Autodesk Fusion 360 part; units mm, degrees
box "BoxPrimitive1" add length 25 width 40 height 25 placed x (0, 0, -1) y (-1, 0, 0) z (0, 1, 0) at (40, 0, 0)
hole "Hole1" at (20, 25, -12.5) direction (0, -1, 0) diameter 8.8 depth 18 tip angle 180
sketch "Sketch2" plane through (40, 0, 0) normal (1, 0, 0) x (0, 0, -1)
  line L0 (0, 25) -> (0, 0)
  line L1 (0, 0) -> (25, 0)
  line L2 (25, 0) -> (25, 25)
  line L3 (25, 25) -> (0, 25)
  line L4 (12.5, 25) -> (12.5, 7) construction
  point P0 (12.5, 9)
  dimension "d9" = 18
  dimension "d10" = 2
hole "Hole2" at (40, 9, -12.5) direction (-1, 0, 0) diameter 2 end through all
hole "Hole3" at (40, 9, -12.5) direction (-1, 0, 0) diameter 6.8 depth 14 tip angle 180
hole "Hole5" at (40, 9, -12.5) direction (-1, 0, 0) diameter 7.2 depth 7.5 tip angle 180
ref_plane "WorkPlane1" through (20, 12.5, -12.5) normal (-1, 0, 0) x (0, 1, 0)
mirror "Mirror1" about plane through (20, 12.5, -12.5) normal (-1, 0, 0) of "Hole3", "Hole5"
ref_plane "WorkPlane2" through (20, 12.5, -12.5) normal (0, 0, 1) x (0, 1, 0)
Could you check a few things on this model? Use its own coordinates, in mm. A direction names the side the tool comes from. Give positions to 0.01 mm unless a question says otherwise; leave off trailing zeros. Loops run counter-clockwise (first coordinate to the right, second up) from the corner with the lowest first, then second, coordinate; pieces in that order, holes last. Notation, with made-up numbers: (-30.5, -1) -> (24.5, -1) arc R27 cw to (24.5, 16) -> close; hole circle Ø2 at (4.25, 70). An arc over 180 degrees is marked (long way). Return JSON: item names as keys, results as strings.
Item 1: If we section it at B-B on y = 9: List the corners of the cut face in (x, z) for me, plus the area to 3 significant figures.
Geometry results:
{"outline": "(0, -25) -> (40, -25) -> (40, -16.1) -> (32.5, -16.1) -> (32.5, -15.9) -> (26, -15.9) -> (26, -13.5) -> (24.28, -13.5) arc R4.4 cw to (15.72, -13.5) -> (14, -13.5) -> (14, -15.9) -> (7.5, -15.9) -> (7.5, -16.1) -> (0, -16.1) -> close; (0, -8.9) -> (7.5, -8.9) -> (7.5, -9.1) -> (14, -9.1) -> (14, -11.5) -> (15.72, -11.5) arc R4.4 cw to (24.28, -11.5) -> (26, -11.5) -> (26, -9.1) -> (32.5, -9.1) -> (32.5, -8.9) -> (40, -8.9) -> (40, 0) -> (0, 0) -> close", "area": "736 mm²"}
Item 2: If we section it at A-A on z = -12.5: Count the separate pieces of the cut face and the enclosed holes in it, plus the area to 3 significant figures.
Geometry results:
{"separate pieces": "3", "enclosed holes": "0", "area": "639 mm²"}
Item 3: We'd pull the mould along Z, two halves only. Please class faces 1 (the flat face through (20, 0, -12)), 2 (the flat face through (20, 12, -25)), 3 (the cylindrical face through (25.13, 8.01, -12.37)), 4 (the cylindrical face through (29.2, 12.32, -11.76)): +Z half, -Z half, draft (parallel to the pull), parting line (faces both ways), or undercut.
Geometry results:
{"face 1": "draft", "face 2": "-Z half", "face 3": "undercut", "face 4": "undercut"}
Item 4: If we section it at C-C on x = 31.5: List the corners of the cut face in (y, z) for me, plus the area to 3 significant figures.
Geometry results:
{"outline": "(0, -25) -> (25, -25) -> (25, 0) -> (0, 0) -> close; hole circle Ø6.8 at (9, -12.5)", "area": "589 mm²"}
Item 5: I need wall thicknesses on L1, parallel to Y at x = 14.6, z = -12.5; L2, parallel to X at y = 10.5, z = -12.5; L3, parallel to Z at x = 35.5, y = 9. Which ranges of each line are inside material? Lowest first, please. Write a range as from..to.
Geometry results:
{"L1": "y = 0..8, 10..25", "L2": "x = 14..15.6, 24.4..26", "L3": "z = -25..-16.1, -8.9..0"}
Item 6: I'm going to push flat-ended pins straight in: pin 1 (9 mm diameter, centred on y = 9, z = -12.5, fed in from +X); pin 2 (2.5 mm diameter, centred on x = 20.5, z = -12, fed in from +Y); pin 3 (2 mm diameter, centred on y = 7.5, z = -12.5, fed in from +X); pin 4 (3 mm diameter, centred on y = 9, z = -12.5, fed in from -X). Where does each tip first touch, or does it pass through?
Geometry results:
{"pin 1": "stops at x = 40", "pin 2": "stops at y = 7", "pin 3": "stops at x = 26", "pin 4": "stops at x = 14"}
Item 7: If we section it at D-D on x = 20: List the corners of the cut face in (y, z) for me, plus the area to 3 significant figures.
Geometry results:
{"outline": "(0, -25) -> (25, -25) -> (25, -16.9) -> (7, -16.9) -> (7, -8.1) -> (25, -8.1) -> (25, 0) -> (0, 0) -> close", "area": "467 mm²"}
Item 8: Which directions (+Z, -Z, +X, -X, +Y, -Y) give clear straight access to the entire face, cutting with the end or side of a thin tool? Please do faces 5 (the flat face through (26, 10.5, -12.5)), 6 (the cylindrical face through (18.678, 15.874, -8.303)), 7 (the cylindrical face through (10.8, 5.68, -11.76)).
Geometry results:
{"face 5": "+X", "face 6": "+Y", "face 7": "-X"}
